Autodesk Inventor part; units mm, degrees
ref_plane "YZ Plane" through (0, 0, 0) normal (1, 0, 0) x (0, 1, 0)
ref_plane "XZ Plane" through (0, 0, 0) normal (0, 1, 0) x (-1, 0, 0)
ref_plane "XY Plane" through (0, 0, 0) normal (0, 0, 1) x (1, 0, 0)
sketch "スケッチ5" plane through (0, 0, 0) normal (0, 0, 1) x (1, 0, 0)
  line L0 (-16, 16) -> (16, 16)
  line L1 (16, 16) -> (16, -16)
  line L2 (16, -16) -> (-16, -16)
  line L3 (-16, -16) -> (-16, 16)
  line L4 (-16, 16) -> (16, -16) construction
  line L5 (16, 16) -> (-16, -16) construction
  line L6 (14.4, 14.4) -> (-14.4, 14.4)
  line L7 (-14.4, 14.4) -> (-14.4, -14.4)
  line L8 (-14.4, -14.4) -> (14.4, -14.4)
  line L9 (14.4, -14.4) -> (14.4, 14.4)
  point P0 (0, 0)
  dimension "d15" = 32
  dimension "d16" = 32
  dimension "d17" = 1.6
extrude "押し出し3" add sketch "スケッチ5" against normal blind 50
sketch "スケッチ6" plane through (0, 0, 0) normal (1, 0, 0) x (0, 1, 0)
  circle A0 centre (0, 0) radius 13.6
  dimension "d20" = 27.2
extrude "押し出し4" cut sketch "スケッチ6" along normal mid plane 32
sketch "スケッチ7" plane through (0, 0, 0) normal (1, 0, 0) x (0, 1, 0)
  line L0 (16, -50) -> (-16, -50)
  circle A0 centre (0, -38) radius 6
  point P0 (0, 0)
  dimension "d23" = 12
  dimension "d24" = 12
extrude "押し出し5" cut sketch "スケッチ7" along normal mid plane 30
properties part number "左右に飛び出すパイプ"
Could you check a few things on this model? Use its own coordinates, in mm. A direction names the side the tool comes from. Give positions to 0.01 mm unless a question says otherwise; leave off trailing zeros. Order: outer loops, then holes, each group sorted by start corner. A loop starts at its lowest first (then second) coordinate and runs counter-clockwise, first axis right, second up.
Item 1: If we section it at D-D, the plane z = -12: Write out the boundary of the cut face in (x, y), plus the area to 3 significant figures.
Item 2: For faces 1 (the face through (0, -14.4, -25)), 2 (the face through (0, 15, 0)), 3 (the face through (15, 0, -38)), which set-ups out of +Z, -Z, +X, -X, +Y, -Y let a thin tool reach every point of the face, with its end or its side?
Item 3: If we section it at B-B, the plane x = -4: Write out the boundary of the cut face in (y, z), plus the area to 3 significant figures.
Item 4: If we section it at A-A, the plane y = -12: Write out the boundary of the cut face in (x, z).
Item 5: I need wall thicknesses on line 1 (X direction, y = -9.5, z = -36.5); line 2 (Z direction, x = -14.7, y = 0). Which ranges of each line are inside material? Lowest first, please.
Item 6: If we section it at C-C, the plane z = -46: Write out the boundary of the cut face in (x, y), plus the area to 3 significant figures.
Item 7: If we mould it in two halves opening along X, with no side actions, what happens to faces 4 (the face through (0, 14.4, -25)), 5 (the face through (0, -15, 0)), 6 (the face through (16, 0, -30)), 7 (the face through (-16, 0, -30))? For each: pulls with the +X half, pulls with the -X half, needs draft (parallel to the pull), parting line crosses it, or undercut.
Values:
1. outline: (-16, -16) - (16, -16) - (16, -6.4) - (14.4, -6.4) - (14.4, -14.4) - (-14.4, -14.4) - (-14.4, -6.4) - (-16, -6.4) - close; (-16, 6.4) - (-14.4, 6.4) - (-14.4, 14.4) - (14.4, 14.4) - (14.4, 6.4) - (16, 6.4) - (16, 16) - (-16, 16) - close
1. area: 154 mm2
2. face 1: +Z, -Z
2. face 2: +Z, +X, -X, +Y, -Y
2. face 3: none
3. outline: (-16, -50) - (-14.4, -50) - (-14.4, 0) - (-16, 0) - close; (14.4, -50) - (16, -50) - (16, 0) - (14.4, 0) - close
3. area: 160 mm2
4. outline: (-16, -50) - (-14.4, -50) - (-14.4, -6.4) - (-16, -6.4) - close; (14.4, -50) - (16, -50) - (16, -6.4) - (14.4, -6.4) - close
5. line 1: x = -16 to -14.4, 14.4 to 16
5. line 2: z = -50 to -44, -32 to -13.6
6. outline: (-16, -16) - (16, -16) - (16, 16) - (-16, 16) - close; hole (-14.4, -14.4) - (14.4, -14.4) - (14.4, 14.4) - (-14.4, 14.4) - close
6. area: 195 mm2
7. face 4: undercut
7. face 5: needs draft
7. face 6: pulls with the +X half
7. face 7: pulls with the -X half
